Can you work these out from the model? Positions are in its coordinate system, mm. A direction names the side the tool comes from. Give positions to 0.01 mm unless a question says otherwise; leave off trailing zeros. Write each loop counter-clockwise with the first axis right and the second up, starting at its lowest first coordinate (ties: lowest second). Pieces come first, ordered by that corner, then holes. Notation, with made-up numbers: (79.5, 1.25) - (88.5, 1.25) arc R13 cw to (88.5, 14.25) - close; hole circle Ø11 at (86, 23). An arc over 180 degrees is marked (long way). Use a Markdown table: item, result. Add a question column.
```python
from build123d import *

# Parameters (mm, degrees)
F0_R     = 4
F0_R_2   = 1.5
F1_DEPTH = 15
F3_DEPTH = 1.5
F5_DEPTH = 1.5


with BuildPart() as f1:
    # F0 (on Right) → F1 (new body)
    with BuildSketch(Plane.YZ):
        Circle(F0_R)
        Circle(F0_R_2, mode=Mode.SUBTRACT)
    extrude(amount=F1_DEPTH)

    # F2 (on Front) → F3 (join, symmetric)
    with BuildSketch(Plane.XZ):
        with BuildLine():
            Line((14.70626425, -3), (0, -3))
            Line((0, -3), (3.3842294856, -12.8433583514))
            ThreePointArc((3.3842294856, -12.8433583514), (7.9879322575, -16.0413339461), (12.4233677026, -12.6137926218))
            Line((12.4233677026, -12.6137926218), (10.6424884871, -11.2477112561))
            ThreePointArc((10.6424884871, -11.2477112561), (5.979534847, -9.5192649707), (10.8988873674, -10.2477112561))
            Line((10.8988873674, -10.2477112561), (13.2192947992, -9.9418605826))
            Line((13.2192947992, -9.9418605826), (14.70626425, -3))
        make_face()
    extrude(amount=F3_DEPTH, both=True)

    # F4 (on Front) → F5 (join)
    with BuildSketch(Plane.XZ):
        with BuildLine():
            Line((0, 7), (0, 3))
            Line((0, 3), (15, 3))
            Line((15, 3), (15, 7))
            ThreePointArc((15, 7), (14.4142135624, 8.4142135624), (13, 9))
            Line((13, 9), (2, 9))
            ThreePointArc((2, 9), (0.5857864376, 8.4142135624), (0, 7))
        make_face()
    extrude(amount=F5_DEPTH)


solid = f1.part
```
Q1. Suppose I cut it at B-B (x = 7). Please give me the cut outline in (y, z).
Q2. Suppose I cut it at C-C (y = -1.25). Please give me the cut outline in (x, z), and give its area (3 significant figures).
Q3. If we mould it in two halves opening along X, with no side actions, what happens to faces 6 (the cylindrical face through (5.956, -0.021, -9.619)), 7 (the flat face through (0, 0, 2)), 8 (the flat face through (15, 0.9, 1.4))? For each: released by +X, released by -X, zero draft, split by the parting line, or undercut.
Q4. Suppose I cut it at A-A (z = 0). Please give me the cut outline in (x, y).
Q5. Suppose I cut it at D-D (x = 2.5). Please give me the cut outline in (y, z).
Q6. I'm going to push flat-ended pins straight in: P1, Ø6, axis at x = 9, z = -8.5, coming from the +Y side; P2, Ø6, axis at x = 8, z = -11.5, coming from the -Y side; P3, Ø2.5, axis at x = 6, z = 5.5, coming from the +Y side; P4, Ø4, axis at x = 11, y = -2.5, coming from the +Z side. Where does each tip first touch, or does it pass through?
Q7. On a 3-axis mill with a long thin cutter (end or side, diameter ignored), from which of +Z, -Z, +X, -X, +Y, -Y can I reach the whole of each face in a straight line? I mean faces 1 (the flat face through (7, 0, 7)), 2 (the flat face through (7, 1.5, -7)), 3 (the flat face through (11.545, -0.021, -11.94)), 4 (the flat face through (7, -1.5, 6)), 5 (the flat face through (7, -1.5, -7)). Say none if no direction works.
Q8. If I drill on probe 1 along Z at (x, y) = (10.5, -0.5); probe 2 along Z at (x, y) = (6.5, -0.75); probe 3 along Y at (x, z) = (3.5, -9.75), over which ranges is the centre line in solid material (lowest first)? Write a range as [from, to].
Derived:
| question | item | result |
|---|---|---|
| 1 | outline | (-1.5, -15.96) - (1.5, -15.96) - (1.5, -12.21) - (-1.5, -12.21) - close; (-1.5, -8.07) - (1.5, -8.07) - (1.5, -3.71) arc R4 ccw to (0, 4) - (0, 9) - (-1.5, 9) - (-1.5, 3.71) arc R4 ccw to (-1.5, -3.71) - close; hole circle Ø3 at (0, 0) |
| 2 | outline | (0, -3.8) - (0.27, -3.8) - (3.38, -12.84) arc R4.74 ccw to (12.42, -12.61) - (10.64, -11.25) arc R2.5 cw (long way) to (10.9, -10.25) - (13.22, -9.94) - (14.53, -3.8) - (15, -3.8) - (15, -0.83) - (0, -0.83) - close; (0, 0.83) - (15, 0.83) - (15, 7) arc R2 ccw to (13, 9) - (2, 9) arc R2 ccw to (0, 7) - close |
| 2 | area | 269 mm² |
| 3 | face 6 | undercut |
| 3 | face 7 | released by -X |
| 3 | face 8 | released by +X |
| 4 | outline | (0, -4) - (15, -4) - (15, -1.5) - (0, -1.5) - close; (0, 1.5) - (15, 1.5) - (15, 4) - (0, 4) - close |
| 5 | outline | (-1.5, -10.27) - (1.5, -10.27) - (1.5, -3.71) arc R4 ccw to (0, 4) - (0, 9) - (-1.5, 9) - (-1.5, 3.71) arc R4 ccw to (-1.5, -3.71) - close; hole circle Ø3 at (0, 0) |
| 6 | P1 | y = 1.5 |
| 6 | P2 | y = -1.5 |
| 6 | P3 | y = 0 |
| 6 | P4 | z = 9 |
| 7 | face 1 | +Z, +X, -X, +Y |
| 7 | face 2 | -Z, +X, -X, +Y |
| 7 | face 3 | +X, +Y, -Y |
| 7 | face 4 | +Z, +X, -X, -Y |
| 7 | face 5 | -Z, +X, -X, -Y |
| 8 | probe 1 | [-15.24, -11.5], [-8.78, -1.41], [1.41, 9] |
| 8 | probe 2 | [-15.84, -11.76], [-8.52, -1.3], [1.3, 9] |
| 8 | probe 3 | [-1.5, 1.5] |
